Geometry: final body of the model. Coordinates: model frame, mm. Face numbers are marked on the shaded views. Give positions to 0.01 mm unless a question says otherwise; leave off trailing zeros. Write each loop counter-clockwise with the first axis right and the second up, starting at its lowest first coordinate (ties: lowest second). Pieces come first, ordered by that corner, then holes.
from build123d import *

# Parameters (mm, degrees)
BOSS_EXTRUDE1_DEPTH = 127
SKETCH2_W           = 31.75
SKETCH2_H           = 38.1
CUT_EXTRUDE1_DEPTH  = 134.953396747
SKETCH3_W           = 76.2
SKETCH3_H           = 31.75
CUT_EXTRUDE2_DEPTH  = 134.953396747
CUT_EXTRUDE3_REACH  = 135.953
SKETCH4_R           = 2.54


with BuildPart() as part:
    # Sketch1 → Boss-Extrude1 (new, symmetric)
    with BuildSketch(Plane.XY):
        Polygon((19.05, 19.05), (-19.05, 19.05), (-19.05, -19.05), (19.05, -19.05), (19.05, -15.875), (-15.875, -15.875), (-15.875, 15.875), (19.05, 15.875), align=None)
    extrude(amount=BOSS_EXTRUDE1_DEPTH, both=True)

    # Sketch2 → Cut-Extrude1 (cut, through all)
    with BuildSketch(Plane(origin=(0, 19.05, 0), x_dir=(1, 0, 0), z_dir=(0, 1, 0))):
        with Locations((3.175, 0)):
            Rectangle(SKETCH2_W, SKETCH2_H)
    extrude(amount=-CUT_EXTRUDE1_DEPTH, mode=Mode.SUBTRACT)

    # Sketch3 → Cut-Extrude2 (cut, through all)
    with BuildSketch(Plane.ZY.offset(19.05)):
        Rectangle(SKETCH3_W, SKETCH3_H)
    extrude(amount=-CUT_EXTRUDE2_DEPTH, mode=Mode.SUBTRACT)

    # Sketch4 → Cut-Extrude3 (cut, up to next)
    with BuildSketch(Plane(origin=(0, 19.05, 0), x_dir=(1, 0, 0), z_dir=(0, 1, 0)), mode=Mode.PRIVATE) as cut_extrude3_sk1:
        with Locations(Location((0, -50.8, 0), (0, 0, 180))):
            Circle(SKETCH4_R)
    cut_extrude3_tool1 = extrude(cut_extrude3_sk1.sketch, amount=-CUT_EXTRUDE3_REACH, mode=Mode.PRIVATE) & part.part
    cut_extrude3 = cut_extrude3_tool1.solids().sort_by_distance((0, 19.05, 50.8))[0]
    add(cut_extrude3, mode=Mode.SUBTRACT)

    # Mirror1: Cut-Extrude3 across plane
    add(cut_extrude3.mirror(Plane.XY), mode=Mode.SUBTRACT)


solid = part.part
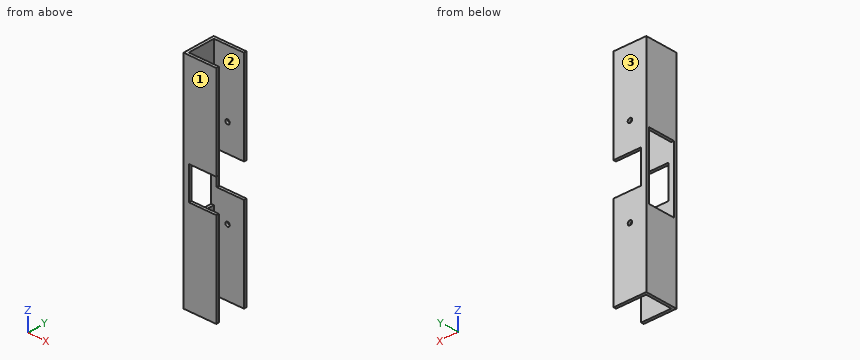
Q1. Section B-B on z = -24.5. Output: boundary loops of the cut face in (x, y) (3 decimals), plus the area to 3 significant figures.
Filled sheet:
outline: (-19.05, -19.05) - (19.05, -19.05) - (19.05, -15.875) - (-19.05, -15.875) - close; (-19.05, 15.875) - (19.05, 15.875) - (19.05, 19.05) - (-19.05, 19.05) - close
area: 242 mm2
Q2. Pull-direction query (Y, two-part tool) for the marked faces 1, 2 and 3; classes: released by +Y, released by -Y, zero draft, split by the parting line, or undercut.
Filled sheet:
face 1: released by -Y
face 2: undercut
face 3: released by +Y
Q3. Pin query (flat end, axial travel): P1, Ø4.5, axis at x = 0, z = -50.8, coming from the +Y side (3 decimals); P2, Ø2.5, axis at y = -17, z = -5.5, coming from the +X side; P3, Ø2, axis at y = -8, z = -41.5, coming from the +X side (3 decimals). Return the tip coordinate at first contact, or that it passes through.
Filled sheet:
P1: stops at y = -15.875
P2: stops at x = -12.7
P3: stops at x = -15.875
Q4. Section D-D on z = 2. Output: boundary loops of the cut face in (x, y) (3 decimals), plus the area to 3 significant figures.
Filled sheet:
outline: (-19.05, -19.05) - (-12.7, -19.05) - (-12.7, -15.875) - (-19.05, -15.875) - close; (-19.05, 15.875) - (-12.7, 15.875) - (-12.7, 19.05) - (-19.05, 19.05) - close
area: 40.3 mm2
Q5. Ray query, line 1 along Z through (x, y) = (0, 17.75); line 2 along Y through (x, z) = (11.5, -115) (3 decimals). Return the intervals inside material, ascending.
Filled sheet:
line 1: z = -127 to -53.34, -48.26 to -19.05, 19.05 to 48.26, 53.34 to 127
line 2: y = -19.05 to -15.875, 15.875 to 19.05
Q6. Section C-C on z = 109.5. Output: boundary loops of the cut face in (x, y) (3 decimals).
Filled sheet:
outline: (-19.05, -19.05) - (19.05, -19.05) - (19.05, -15.875) - (-15.875, -15.875) - (-15.875, 15.875) - (19.05, 15.875) - (19.05, 19.05) - (-19.05, 19.05) - close
Q7. Section A-A on x = -7. Output: boundary loops of the cut face in (y, z) (3 decimals), plus the area to 3 significant figures.
Filled sheet:
outline: (-19.05, -127) - (-15.875, -127) - (-15.875, -19.05) - (-19.05, -19.05) - close; (-19.05, 19.05) - (-15.875, 19.05) - (-15.875, 127) - (-19.05, 127) - close; (15.875, -127) - (19.05, -127) - (19.05, -19.05) - (15.875, -19.05) - close; (15.875, 19.05) - (19.05, 19.05) - (19.05, 127) - (15.875, 127) - close
area: 1,370 mm2
